Design review of the part built by this model. Coordinates are the model's own, in mm. Coordinates: 2 decimals unless noted, no trailing zeros. Write each loop counter-clockwise with the first axis right and the second up, starting at its lowest first coordinate (ties: lowest second). Pieces come first, ordered by that corner, then holes. Notation, with made-up numbers: (18.5, 59) - (32.5, 59) arc R35 ccw to (32.5, 93) - close; hole circle Ø1 at (11, -14). An arc over 180 degrees is marked (long way). One line per item, written item: value.
from build123d import *

# Parameters (mm, degrees)
BOSS_EXTRUDE1_DEPTH    = 3.175
F_10_CLEARANCE_HOLE1_D = 4.9784
SKETCH8_R              = 9.525
CUT_EXTRUDE1_DEPTH     = 305.646421585


with BuildPart() as part:
    # Sketch2 → Boss-Extrude1 (new body)
    with BuildSketch(Plane.XY):
        Polygon((75.605515224, 191.084223429), (41.804664545, 295.09857273), (4.854209552, 283.091029346), (4.854209552, 203.901454104), align=None)
    extrude(amount=BOSS_EXTRUDE1_DEPTH)

    # #10 Clearance Hole1 (through all)
    with Locations(Plane.XY.offset(3.175)):
        with Locations((32.740251946, 283.138719963), (59.435154755, 200.980257064), (12.7, 238.125), (12.7, 212.725), (14.622625311, 277.25194622), (14.622625311, 258.20194622)):
            Hole(F_10_CLEARANCE_HOLE1_D / 2)

    # Sketch8 → Cut-Extrude1 (cut, through all)
    with BuildSketch(Plane(origin=(0, 0, 0), x_dir=(-1, 0, 0), z_dir=(0, 0, -1))):
        with Locations((-50.8, 225.425)):
            Circle(SKETCH8_R)
    extrude(amount=-CUT_EXTRUDE1_DEPTH, mode=Mode.SUBTRACT)


solid = part.part
1. Consider section D-D, the plane y = 253.5. Write out the cut boundary in (x, z) (3 decimals).
Answer block:
outline: (4.854, 0) - (55.323, 0) - (55.323, 3.175) - (4.854, 3.175) - close
2. Mouldability with a two-part tool opening along Y and no side actions: class faces 1 (the face through (59.76, 203.45, 1.57)), 2 (the face through (23.59, 289.18, 1.57)), 3 (the face through (4.854, 244, 2)), 4 (the face through (39.735, 197.583, 1.565)) as released by +Y, released by -Y, zero draft, split by the parting line, or undercut.
Answer block:
face 1: undercut
face 2: released by +Y
face 3: zero draft
face 4: released by -Y
3. Consider section C-C, the plane x = 33. Write out the cut boundary in (y, z) (3 decimals).
Answer block:
outline: (198.803, 0) - (280.663, 0) - (280.663, 3.175) - (198.803, 3.175) - close; (285.614, 0) - (292.237, 0) - (292.237, 3.175) - (285.614, 3.175) - close
4. Consider section B-B, the plane z = 2. Write out the cut boundary in (x, y) (3 decimals).
Answer block:
outline: (4.854, 203.901) - (75.606, 191.084) - (41.805, 295.099) - (4.854, 283.091) - close; hole circle Ø4.978 at (12.7, 212.725); hole circle Ø4.978 at (12.7, 238.125); hole circle Ø4.978 at (14.623, 258.202); hole circle Ø4.978 at (14.623, 277.252); hole circle Ø4.978 at (32.74, 283.139); hole circle Ø19.05 at (50.8, 225.425); hole circle Ø4.978 at (59.435, 200.98)
5. Wall thickness on line 1 along X through (y, z) = (230, 0.8); line 2 along X through (y, z) = (214, 0.4); line 3 along Y through (x, z) = (36, 1.05): over which ranges is each line inside the solid? List them lowest first.
Answer block:
line 1: x = 4.85 to 42.45, 59.15 to 62.96
line 2: x = 4.85 to 10.56, 14.84 to 68.16
line 3: y = 198.26 to 293.21
6. Insertion check: pin 1 Ø8 at (x, y) = (59.44, 200.98) entering from -Z; pin 2 Ø1.5 at (y, z) = (271, 1) entering from +X. Each pin has a flat end and moves straight along its axis. Give the tip position at first contact, or say it passes through.
Answer block:
pin 1: stops at z = 0
pin 2: stops at x = 49.88
7. Consider section A-A, the plane x = 55. Write out the cut boundary in (y, z) (3 decimals).
Answer block:
outline: (194.817, 0) - (216.876, 0) - (216.876, 3.175) - (194.817, 3.175) - close; (233.974, 0) - (254.493, 0) - (254.493, 3.175) - (233.974, 3.175) - close
